from build123d import *

# Parameters (mm, degrees)
F0_R     = 15.875
F0_R_2   = 11.1125
F1_DEPTH = 6.35
F2_SIZE  = 1.5875


with BuildPart() as f1:
    # F0 (on Front) → F1 (new body)
    with BuildSketch(Plane.XZ):
        Circle(F0_R)
        Circle(F0_R_2, mode=Mode.SUBTRACT)
    extrude(amount=F1_DEPTH)

    # F2
    f2_edges = [f1.edges().sort_by_distance(p)[0] for p in [
        (-15.875, -6.35, 0),
    ]]
    chamfer(f2_edges, length=F2_SIZE)

    # F5: sweep along a path in F3
    with BuildLine(Plane(origin=(0, 0, 0), x_dir=(-1, 0, 0), z_dir=(0, 1, 0))) as f5_path:
        CenterArc((0, 0), 11.90625, 0, 360)
    # F4 (on Right) → F5 (sweep, cut)
    with BuildSketch(Plane.YZ):
        with BuildLine():
            ThreePointArc((1.5875, 13.49375), (1.122532, 14.616282), (0, 15.08125))
            Line((0, 15.08125), (0, 11.90625))
            ThreePointArc((0, 11.90625), (1.122532, 12.371218), (1.5875, 13.49375))
        make_face()
        with BuildLine():
            Line((0, 11.90625), (0, 15.08125))
            ThreePointArc((0, 15.08125), (-1.5875, 13.49375), (0, 11.90625))
        make_face()
    sweep(path=f5_path.line, mode=Mode.SUBTRACT)


solid = f1.part
Can you work these out from the model? Positions are in its coordinate system, mm. Give positions to 0.01 mm unless a question says otherwise; leave off trailing zeros. Return JSON: item names as keys, results as strings.
1. I want a section at D-D on y = -1. Give the number of separate pieces and of enclosed holes in the cut face, and give its area (3 significant figures).
Output values:
{"separate pieces": "2", "enclosed holes": "2", "area": "195 mm²"}
2. If I drill on line 1 (Z direction, x = 0, y = -2.75) (1 decimal); line 2 (Z direction, x = 0, y = -1.25) (1 decimal); line 3 (Z direction, x = -5, y = -5.5), over which ranges is the centre line in solid material (lowest first)?
Output values:
{"line 1": "z = -15.9 to -11.1, 11.1 to 15.9", "line 2": "z = -15.9 to -14.5, -12.5 to -11.1, 11.1 to 12.5, 14.5 to 15.9", "line 3": "z = -14.29 to -9.92, 9.92 to 14.29"}
3. I'm going to push flat-ended pins straight in: pin 1 Ø3 at (y, z) = (-4, 3.5) entering from -X; pin 2 Ø1 at (x, z) = (-1, -9) entering from +Y. Where does each tip first touch, or does it pass through?
Output values:
{"pin 1": "stops at x = -15.75", "pin 2": "passes through"}
4. We'd pull the mould along X, two halves only. Please class faces 1 (the face through (10.6, -3.13, 3.34)), 2 (the face through (-3.441, -2.348, -15.497)), 3 (the face through (-9, -6.35, -7)): +X half, -X half, draft (parallel to the pull), parting line (faces both ways), or undercut.
Output values:
{"face 1": "undercut", "face 2": "parting line", "face 3": "draft"}
